Geometry: see drawing. Coordinates: mm, zero at the bounding-box minimum. Coordinates: 2 decimals unless noted, no trailing zeros. Order: outer loops, then holes, each group sorted by start corner. A loop starts at its lowest first (then second) coordinate and runs counter-clockwise, first axis right, second up. Notation, with made-up numbers: (-24.75, 80) -> (33.25, 80) arc R23 ccw to (33.25, 114) -> close; hole circle Ø5 at (-12, 35.25). An arc over 180 degrees is marked (long way). Use one line per item in the form item = value.
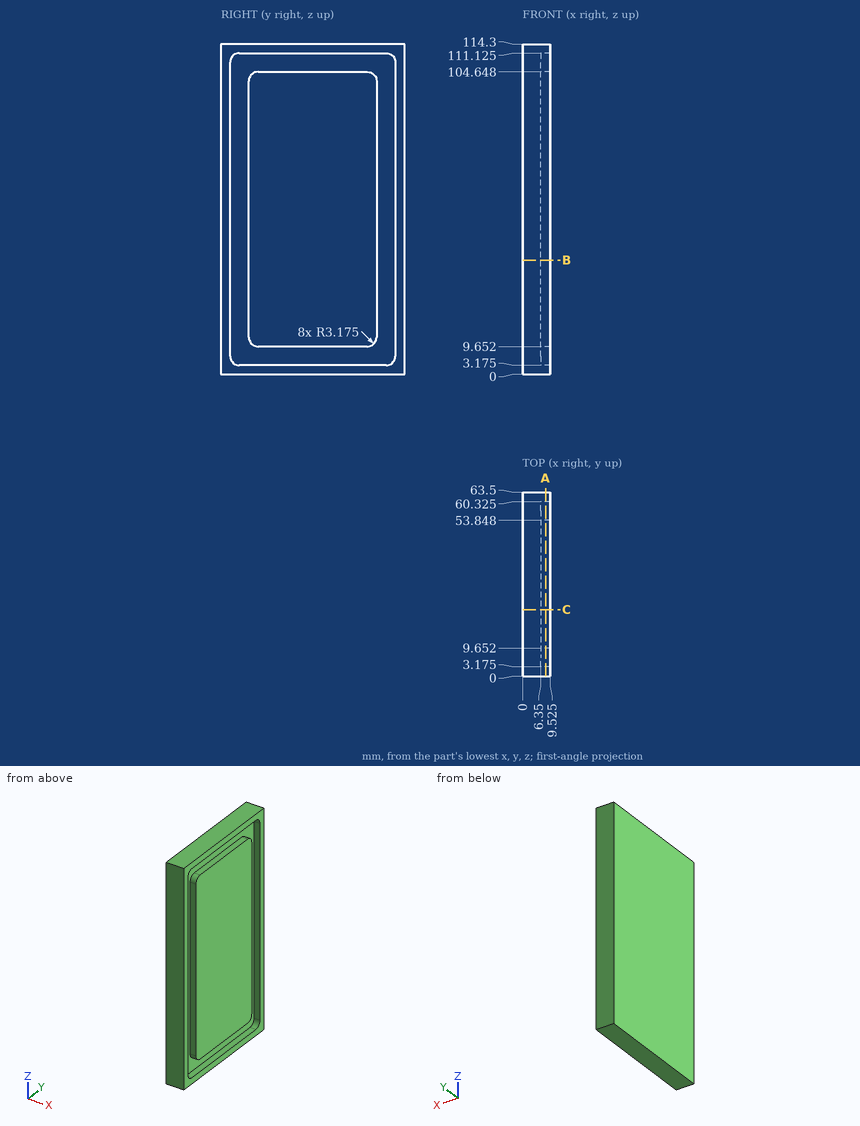
1) Section C-C, the plane y = 23. Output: boundary loops of the cut face in (x, z) (3 decimals).
Results found:
outline = (0, 0) -> (9.525, 0) -> (9.525, 3.175) -> (6.35, 3.175) -> (6.35, 9.652) -> (9.525, 9.652) -> (9.525, 104.648) -> (6.35, 104.648) -> (6.35, 111.125) -> (9.525, 111.125) -> (9.525, 114.3) -> (0, 114.3) -> close
2) Section B-B, the plane z = 39.5. Output: boundary loops of the cut face in (x, y) (3 decimals).
Results found:
outline = (0, 0) -> (9.525, 0) -> (9.525, 3.175) -> (6.35, 3.175) -> (6.35, 9.652) -> (9.525, 9.652) -> (9.525, 53.848) -> (6.35, 53.848) -> (6.35, 60.325) -> (9.525, 60.325) -> (9.525, 63.5) -> (0, 63.5) -> close
3) Section A-A, the plane x = 8. Output: boundary loops of the cut face in (y, z) (3 decimals).
Results found:
outline = (0, 0) -> (63.5, 0) -> (63.5, 114.3) -> (0, 114.3) -> close; (9.652, 12.827) arc R3.175 ccw to (12.827, 9.652) -> (50.673, 9.652) arc R3.175 ccw to (53.848, 12.827) -> (53.848, 101.473) arc R3.175 ccw to (50.673, 104.648) -> (12.827, 104.648) arc R3.175 ccw to (9.652, 101.473) -> close; hole (3.175, 6.35) arc R3.175 ccw to (6.35, 3.175) -> (57.15, 3.175) arc R3.175 ccw to (60.325, 6.35) -> (60.325, 107.95) arc R3.175 ccw to (57.15, 111.125) -> (6.35, 111.125) arc R3.175 ccw to (3.175, 107.95) -> close
4) Contact query for a flat-ended pin moving along its axis: P1, Ø2, axis at x = 4, z = 94.5, coming from the -Y side. Output: stop coordinate, or through.
Results found:
P1 = 0
5) Material intervals for probe 1 along Z at (x, y) = (6.75, 44.5) (3 decimals); probe 2 along Y at (x, z) = (6.75, 37) (3 decimals); probe 3 along X at (y, z) = (3.5, 31), sorted ascending. Write a range as from..to.
Results found:
probe_1 = 0..3.175, 9.652..104.648, 111.125..114.3
probe_2 = 0..3.175, 9.652..53.848, 60.325..63.5
probe_3 = 0..6.35
